```python
from build123d import *

# Parameters (mm, degrees)
SKETCH1_R           = 32.5
BOSS_EXTRUDE1_DEPTH = 2
SKETCH2_R           = 32.5
BOSS_EXTRUDE2_DEPTH = 13
SKETCH6_W           = 71.390071862
SKETCH6_H           = 35.774890597
CUT_EXTRUDE4_DEPTH  = 13
SNAP_START          = 30
SNAP_HOOK1_DEPTH    = 2
SNAP_START_2        = 6.002601726
SNAP_HOOK1_2_DEPTH  = 4.628893351
SNAP_START_3        = 27
SNAP_HOOK1_3_DEPTH  = 3


with BuildPart() as part:
    # Sketch1 → Boss-Extrude1 (new body)
    with BuildSketch(Plane(origin=(0, 0, 0), x_dir=(1, 0, 0), z_dir=(0, 1, 0))):
        with Locations(Location((0, 0, 0), (0, 0, 270))):
            Circle(SKETCH1_R)
    extrude(amount=BOSS_EXTRUDE1_DEPTH)

    # Sketch2 → Boss-Extrude2 (add)
    with BuildSketch(Plane(origin=(0, 2, 0), x_dir=(1, 0, 0), z_dir=(0, 1, 0))):
        with Locations(Location((0, 0, 0), (0, 0, 270))):
            Circle(SKETCH2_R)
        with BuildLine():
            Line((2.6, -27.125679715), (2.6, -30))
            Line((2.6, -30), (-2.6, -30))
            Line((-2.6, -30), (-2.6, -27.125679715))
            ThreePointArc((-2.6, -27.125679715), (-19.268659787, -19.268659787), (-27.125679715, -2.6))
            Line((-27.125679715, -2.6), (-30, -2.6))
            Line((-30, -2.6), (-30, 2.6))
            Line((-30, 2.6), (-27.125679715, 2.6))
            ThreePointArc((-27.125679715, 2.6), (-19.268659787, 19.268659787), (-2.6, 27.125679715))
            Line((-2.6, 27.125679715), (-2.6, 30))
            Line((-2.6, 30), (2.6, 30))
            Line((2.6, 30), (2.6, 27.125679715))
            ThreePointArc((2.6, 27.125679715), (19.268659787, 19.268659787), (27.125679715, 2.6))
            Line((27.125679715, 2.6), (30, 2.6))
            Line((30, 2.6), (30, -2.6))
            Line((30, -2.6), (27.125679715, -2.6))
            ThreePointArc((27.125679715, -2.6), (19.268659787, -19.268659787), (2.6, -27.125679715))
        make_face(mode=Mode.SUBTRACT)
    extrude(amount=BOSS_EXTRUDE2_DEPTH)

    # Sketch6 → Cut-Extrude4 (cut)
    with BuildSketch(Plane(origin=(0, 15, 0), x_dir=(1, 0, 0), z_dir=(0, 1, 0))):
        with Locations((0.159709333, -17.887445299)):
            Rectangle(SKETCH6_W, SKETCH6_H)
    extrude(amount=-CUT_EXTRUDE4_DEPTH, mode=Mode.SUBTRACT)

    # Snap Hook1: read off the stored shape, not the designer's step
    # Snap Hook1 outline → Snap Hook1 (add)
    with BuildSketch(Plane.YZ.offset(SNAP_START)):
        Polygon((6.317048401, 16), (5.478523933, 0), (11.15557287, 0), (10.317048401, 16), align=None)
    extrude(amount=SNAP_HOOK1_DEPTH)

    # Snap Hook1 2 outline → Snap Hook1 2 (add)
    with BuildSketch(Plane(origin=(0, 0, 0), x_dir=(1, 0, 0), z_dir=(0, 1, 0)).offset(SNAP_START_2)):
        Polygon((30, -16), (30, -10), (28, -10), align=None)
    extrude(amount=SNAP_HOOK1_2_DEPTH)

    # Snap Hook1 3 outline → Snap Hook1 3 (cut)
    with BuildSketch(Plane.YZ.offset(SNAP_START_3)):
        Polygon((6.002601726, 10), (6.317048401, 16), (6.36945618, 17), (6.002601726, 17), align=None)
        Polygon((10.631495077, 17), (10.264640622, 17), (10.317048401, 16), (10.631495077, 10), align=None)
    extrude(amount=SNAP_HOOK1_3_DEPTH, mode=Mode.SUBTRACT)


solid = part.part
```
Design review of the part built by this model. Coordinates are the model's own, in mm. A direction names the side the tool comes from. Give positions to 0.01 mm unless a question says otherwise; leave off trailing zeros. Write each loop counter-clockwise with the first axis right and the second up, starting at its lowest first coordinate (ties: lowest second). Pieces come first, ordered by that corner, then holes. Notation, with made-up numbers: (59.25, -4) -> (69.25, -4) arc R18 ccw to (69.25, 0) -> close; hole circle Ø6 at (-16.75, 47). An arc over 180 degrees is marked (long way). Answer in a Markdown table with one row per item.
(1) Mouldability with a two-part tool opening along X and no side actions: class faces 4 (the cylindrical face through (19.082, 8.409, -19.454)), 5 (the flat face through (32, 8, 8)), 6 (the flat face through (31, 8, 16)), 7 (the flat face through (-30, 8, -1)) as +X half, -X half, draft (parallel to the pull), parting line (faces both ways), or undercut.
Results:
| item | result |
|---|---|
| face 4 | undercut |
| face 5 | +X half |
| face 6 | draft |
| face 7 | undercut |
(2) To check wall thickness, follow probe 1 along Y at (x, z) = (19.5, 6.5); probe 2 along X at (y, z) = (7.5, -2); probe 3 along X at (y, z) = (3, -3). State the ranges of each line that lie inside material, in increasing order.
Results:
| item | result |
|---|---|
| probe 1 | 0 to 2 |
| probe 2 | -32.44 to -30, 30 to 32.44 |
| probe 3 | -32.36 to -27.08, 27.08 to 32.36 |
(3) Clearance check with flat-ended pins moving along their axes: pin 1 (1.5 mm diameter, centred on x = -15.5, z = 0.5, fed in from +Y); pin 2 (1.5 mm diameter, centred on x = 23.5, y = 12, fed in from +Z); pin 3 (2.5 mm diameter, centred on y = 7, z = -28.5, fed in from +X). State where each tip first meets the part, or that it passes through.
Results:
| item | result |
|---|---|
| pin 1 | y = 2 |
| pin 2 | z = -12.43 |
| pin 3 | x = 17.71 |
(4) Consider section B-B (z = -19). State the section outline as (x, y) points, then the cut area to 3 significant figures.
Results:
| item | result |
|---|---|
| outline | (-26.37, 0) -> (26.37, 0) -> (26.37, 15) -> (19.53, 15) -> (19.53, 2) -> (-19.53, 2) -> (-19.53, 15) -> (-26.37, 15) -> close |
| area | 283 mm2 |
(5) Consider section C-C (x = 0). State the section outline as (y, z) points, then the cut area to 4 significant figures.
Results:
| item | result |
|---|---|
| outline | (0, -32.5) -> (15, -32.5) -> (15, -30) -> (2, -30) -> (2, 32.5) -> (0, 32.5) -> close |
| area | 162.5 mm2 |
(6) Consider section D-D (z = -9.5). State the section outline as (x, y) points, then the cut area to 3 significant figures.
Results:
| item | result |
|---|---|
| outline | (-31.08, 0) -> (31.08, 0) -> (31.08, 15) -> (25.54, 15) -> (25.54, 2) -> (-25.54, 2) -> (-25.54, 15) -> (-31.08, 15) -> close |
| area | 268 mm2 |
(7) Consider section A-A (y = 9.25). State the section outline as (x, z) points.
Results:
| item | result |
|---|---|
| outline | (-32.5, 0) arc R32.5 ccw to (32.5, 0) -> (32, 0) -> (32, 16) -> (30, 16) -> (28, 10) -> (30, 10) -> (30, -2.6) -> (27.13, -2.6) arc R27.25 cw to (2.6, -27.13) -> (2.6, -30) -> (-2.6, -30) -> (-2.6, -27.13) arc R27.25 cw to (-27.13, -2.6) -> (-30, -2.6) -> (-30, 0) -> close |
(8) For faces 1 (the flat face through (0, 8, -30)), 2 (the flat face through (30, 8, 2)), 3 (the flat face through (29, 8, 13)), list the 3-axis set-ups (+Z, -Z, +X, -X, +Y, -Y) from which the entire face can be reached by the end or side of a thin tool; tool diameter is ignored.
Results:
| item | result |
|---|---|
| face 1 | +Z, +Y |
| face 2 | +Y |
| face 3 | +Z, -X, +Y |
